Geometry check sheet. Reference: the model listing, model coordinates, mm. A direction names the side the tool comes from. Give positions to 0.01 mm unless a question says otherwise; leave off trailing zeros. Loops run counter-clockwise (first coordinate to the right, second up) from the corner with the lowest first, then second, coordinate; pieces in that order, holes last. Notation, with made-up numbers: (80.25, 60) -> (98.25, 60) arc R11 ccw to (98.25, 80) -> close; hole circle Ø5 at (27.25, -21). An arc over 180 degrees is marked (long way). One line per item, written item: value. Start each with the question number.
(1) Draft check along X on faces 4 (the face through (-36, 12.3, 4)), 5 (the face through (-16, 2, 21.25)). Enter one of: pulls with the +X half, pulls with the -X half, needs draft (parallel to the pull), parting line crosses it, or undercut.
(2) Sectioned sample at A-A, the plane z = -16. Record the cut outline in (x, y), then the cut area to 3 significant figures.
(3) Gauge pin test, flat ends, axial feed: pin 1 Ø8 at (x, z) = (-7, -13.5) entering from +Y; pin 2 Ø1.9 at (x, z) = (-42, -26) entering from +Y; pin 3 Ø4 at (x, z) = (-12.5, 16.5) entering from +Y. Record the tip position at first contact, or that the pin passes through.
(4) Scan lines: line 1 along X through (y, z) = (7.75, -6.5); line 2 along X through (y, z) = (5.5, -26); line 3 along X through (y, z) = (6.75, 4). Record each from-to range of solid material in increasing order. Write a range as from..to.
(5) Sectioned sample at C-C, the plane z = 20. Record the cut outline in (x, y), then the cut area to 3 significant figures.
(6) Tool access check on faces 1 (the face through (45, 12.3, -29)), 2 (the face through (46.44, 11.44, 28.54)), 3 (the face through (16, 5, -24)). Record the directions out of +Z, -Z, +X, -X, +Y, -Y that give a thin tool (end or side, any length) a straight path to the whole face; none if there is none.
(7) Sectioned sample at B-B, the plane y = 3.25. State how many separate pieces and enclosed holes the cut face has, then the cut area to 3 significant figures.
(8) Sectioned sample at D-D, the plane x = -30. Record the cut outline in (y, z), then the cut area to 3 significant figures.
from build123d import *

# Parameters (mm, degrees)
SKETCH1_W           = 96
SKETCH1_H           = 64
BOSS_EXTRUDE1_DEPTH = 10.6
CUT_EXTRUDE1_DEPTH  = 6
SKETCH3_W           = 8.5
SKETCH3_H           = 2.75
CUT_EXTRUDE2_DEPTH  = 59
SKETCH4_R           = 1.6
CUT_EXTRUDE3_DEPTH  = 59.654582089
CHAMFER1_SIZE       = 2
SKETCH5_R           = 2.5
BOSS_EXTRUDE3_DEPTH = 1.7
SKETCH6_R           = 3.6
CUT_EXTRUDE5_DEPTH  = 59.654582089


with BuildPart() as part:
    # Sketch1 → Boss-Extrude1 (new body)
    with BuildSketch(Plane(origin=(0, 0, 0), x_dir=(1, 0, 0), z_dir=(0, 1, 0))):
        Rectangle(SKETCH1_W, SKETCH1_H)
    extrude(amount=BOSS_EXTRUDE1_DEPTH)

    # Sketch2 → Cut-Extrude1 (cut)
    with BuildSketch(Plane(origin=(0, 10.6, 0), x_dir=(1, 0, 0), z_dir=(0, 1, 0))):
        Polygon((-20.5, 18.5), (-20.5, 24), (-12, 24), (-12, 18.5), (-8, 18.5), (-8, 2), (-24.5, 2), (-24.5, 18.5), align=None)
        Polygon((-24.5, -2), (-8, -2), (-8, -18.5), (-12, -18.5), (-12, -24), (-20.5, -24), (-20.5, -18.5), (-24.5, -18.5), align=None)
        Polygon((24.5, -2), (24.5, -18.5), (20.5, -18.5), (20.5, -24), (12, -24), (12, -18.5), (8, -18.5), (8, -2), align=None)
        Polygon((24.5, 2), (8, 2), (8, 18.5), (12, 18.5), (12, 24), (20.5, 24), (20.5, 18.5), (24.5, 18.5), align=None)
    extrude(amount=-CUT_EXTRUDE1_DEPTH, mode=Mode.SUBTRACT)

    # Sketch3 → Cut-Extrude2 (cut, through all)
    with BuildSketch(Plane(origin=(0, 4.6, 0), x_dir=(1, 0, 0), z_dir=(0, 1, 0))):
        with Locations((-16.25, 22.625)):
            Rectangle(SKETCH3_W, SKETCH3_H)
        with Locations((16.25, 22.625)):
            Rectangle(SKETCH3_W, SKETCH3_H)
        with Locations((-16.25, -22.625)):
            Rectangle(SKETCH3_W, SKETCH3_H)
        with Locations((16.25, -22.625)):
            Rectangle(SKETCH3_W, SKETCH3_H)
    extrude(amount=-CUT_EXTRUDE2_DEPTH, mode=Mode.SUBTRACT)

    # Sketch4 → Cut-Extrude3 (cut, through all)
    with BuildSketch(Plane(origin=(0, 10.6, 0), x_dir=(1, 0, 0), z_dir=(0, 1, 0))):
        with Locations(Location((-42, 26, 0), (0, 0, 270))):
            Circle(SKETCH4_R)
        with Locations(Location((42, 26, 0), (0, 0, 90))):
            Circle(SKETCH4_R)
        with Locations(Location((-42, -26, 0), (0, 0, 90))):
            Circle(SKETCH4_R)
        with Locations(Location((42, -4, 0), (0, 0, 270))):
            Circle(SKETCH4_R)
    extrude(amount=-CUT_EXTRUDE3_DEPTH, mode=Mode.SUBTRACT)

    # Chamfer1
    chamfer1_edges = [part.edges().sort_by_distance(p)[0] for p in [
        (42, 10.6, -24.4),
        (-42, 10.6, 27.6),
        (42, 10.6, 2.4),
        (-42, 10.6, -27.6),
    ]]
    chamfer(chamfer1_edges, length=CHAMFER1_SIZE)

    # Sketch5 → Boss-Extrude3 (add)
    with BuildSketch(Plane(origin=(0, 10.6, 0), x_dir=(1, 0, 0), z_dir=(0, 1, 0))):
        with Locations(Location((-44, 28, 0), (0, 0, 39.766388891))):
            Circle(SKETCH5_R)
        with Locations(Location((-36, 28, 0), (0, 0, 90))):
            Circle(SKETCH5_R)
        with Locations(Location((-44, 20, 0), (0, 0, 90))):
            Circle(SKETCH5_R)
        with Locations(Location((-36, 20, 0), (0, 0, 90))):
            Circle(SKETCH5_R)
        with Locations(Location((-44, 12, 0), (0, 0, 90))):
            Circle(SKETCH5_R)
        with Locations(Location((-36, 12, 0), (0, 0, 90))):
            Circle(SKETCH5_R)
        with Locations(Location((-44, 4, 0), (0, 0, 90))):
            Circle(SKETCH5_R)
        with Locations(Location((-36, 4, 0), (0, 0, 90))):
            Circle(SKETCH5_R)
        with Locations(Location((-44, -4, 0), (0, 0, 90))):
            Circle(SKETCH5_R)
        with Locations(Location((-36, -4, 0), (0, 0, 90))):
            Circle(SKETCH5_R)
        with Locations(Location((36, -4, 0), (0, 0, 90))):
            Circle(SKETCH5_R)
        with Locations(Location((44, -4, 0), (0, 0, 90))):
            Circle(SKETCH5_R)
        with Locations(Location((44, 4, 0), (0, 0, 90))):
            Circle(SKETCH5_R)
        with Locations(Location((36, 4, 0), (0, 0, 90))):
            Circle(SKETCH5_R)
        with Locations(Location((36, 12, 0), (0, 0, 90))):
            Circle(SKETCH5_R)
        with Locations(Location((44, 12, 0), (0, 0, 90))):
            Circle(SKETCH5_R)
        with Locations(Location((44, 20, 0), (0, 0, 90))):
            Circle(SKETCH5_R)
        with Locations(Location((36, 20, 0), (0, 0, 90))):
            Circle(SKETCH5_R)
        with Locations(Location((36, 28, 0), (0, 0, 90))):
            Circle(SKETCH5_R)
        with Locations(Location((44, 28, 0), (0, 0, 90))):
            Circle(SKETCH5_R)
        with Locations(Location((-44, -12, 0), (0, 0, 90))):
            Circle(SKETCH5_R)
        with Locations(Location((-36, -12, 0), (0, 0, 90))):
            Circle(SKETCH5_R)
        with Locations(Location((-44, -20, 0), (0, 0, 90))):
            Circle(SKETCH5_R)
        with Locations(Location((-36, -20, 0), (0, 0, 90))):
            Circle(SKETCH5_R)
        with Locations(Location((-44, -28, 0), (0, 0, 129.766388891))):
            Circle(SKETCH5_R)
        with Locations(Location((-36, -28, 0), (0, 0, 90))):
            Circle(SKETCH5_R)
        with Locations(Location((36, -28, 0), (0, 0, 90))):
            Circle(SKETCH5_R)
        with Locations(Location((36, -20, 0), (0, 0, 90))):
            Circle(SKETCH5_R)
        with Locations(Location((36, -12, 0), (0, 0, 90))):
            Circle(SKETCH5_R)
        with Locations(Location((44, -12, 0), (0, 0, 90))):
            Circle(SKETCH5_R)
        with Locations(Location((44, -20, 0), (0, 0, 90))):
            Circle(SKETCH5_R)
        with Locations(Location((44, -28, 0), (0, 0, 90))):
            Circle(SKETCH5_R)
    extrude(amount=BOSS_EXTRUDE3_DEPTH)

    # Sketch6 → Cut-Extrude5 (cut, through all)
    with BuildSketch(Plane(origin=(0, 10.6, 0), x_dir=(1, 0, 0), z_dir=(0, 1, 0))):
        with Locations((-42, 26)):
            Circle(SKETCH6_R)
        with Locations((-42, -26)):
            Circle(SKETCH6_R)
        with Locations((42, -4)):
            Circle(SKETCH6_R)
        with Locations((42, 26)):
            Circle(SKETCH6_R)
    extrude(amount=CUT_EXTRUDE5_DEPTH, mode=Mode.SUBTRACT)


solid = part.part
Calculated:
1. face 4: needs draft
1. face 5: undercut
2. outline: (-48, 0) -> (48, 0) -> (48, 10.6) -> (24.5, 10.6) -> (24.5, 4.6) -> (8, 4.6) -> (8, 10.6) -> (-8, 10.6) -> (-8, 4.6) -> (-24.5, 4.6) -> (-24.5, 10.6) -> (-48, 10.6) -> close
2. area: 820 mm2
3. pin 1: stops at y = 10.6
3. pin 2: passes through
3. pin 3: stops at y = 4.6
4. line 1: x = -48..-24.5, -8..8, 24.5..48
4. line 2: x = -48..-43.6, -40.4..40.4, 43.6..48
4. line 3: x = -48..-24.5, -8..8, 24.5..40.4, 43.6..48
5. outline: (-48, 0) -> (48, 0) -> (48, 10.6) -> (46.5, 10.6) -> (46.5, 12.3) -> (41.5, 12.3) -> (41.5, 10.6) -> (38.5, 10.6) -> (38.5, 12.3) -> (33.5, 12.3) -> (33.5, 10.6) -> (20.5, 10.6) -> (20.5, 4.6) -> (12, 4.6) -> (12, 10.6) -> (-12, 10.6) -> (-12, 4.6) -> (-20.5, 4.6) -> (-20.5, 10.6) -> (-33.5, 10.6) -> (-33.5, 12.3) -> (-38.5, 12.3) -> (-38.5, 10.6) -> (-41.5, 10.6) -> (-41.5, 12.3) -> (-46.5, 12.3) -> (-46.5, 10.6) -> (-48, 10.6) -> close
5. area: 950 mm2
6. face 1: +Z, -Z, +X, -X, +Y
6. face 2: +Y
6. face 3: +Y, -Y
7. separate pieces: 1
7. enclosed holes: 8
7. area: 6,020 mm2
8. outline: (0, -32) -> (10.6, -32) -> (10.6, 32) -> (0, 32) -> close
8. area: 678 mm2
